```python
from build123d import *

# Parameters (mm, degrees)
F0_W     = 114.3
F0_H     = 76.2
F1_DEPTH = 25.4
F2_R     = 5.08
F3_T     = -3.81
F4_R     = 4.953
F5_DEPTH = 25.4
F7_DEPTH = 3.81


with BuildPart() as f1:
    # F0 (on Top) → F1 (new body)
    with BuildSketch(Plane.XY):
        with Locations((57.15, -38.1)):
            Rectangle(F0_W, F0_H)
    extrude(amount=F1_DEPTH)

    # F2
    f2_edges = [f1.edges().sort_by_distance(p)[0] for p in [
        (114.3, 0, 12.7),
        (114.3, -76.2, 12.7),
        (0, 0, 12.7),
        (0, -76.2, 12.7),
    ]]
    fillet(f2_edges, radius=F2_R)

    # F3
    f3_openings = [f1.faces().sort_by_distance(p)[0] for p in [
        (57.15, -38.1, 0),
    ]]
    offset(amount=F3_T, openings=f3_openings)

    # F4 (on face) → F5 (cut)
    with BuildSketch(Plane.YZ.offset(114.3)):
        with Locations((-25.4, 12.7)):
            Circle(F4_R)
    extrude(amount=-F5_DEPTH, mode=Mode.SUBTRACT)

    # F6 (on face) → F7 (join)
    with BuildSketch(Plane.XY.offset(25.4)):
        with BuildLine():
            Line((109.22, 3.937), (5.08, 3.937))
            ThreePointArc((5.08, 3.937), (-1.295982, 1.295982), (-3.937, -5.08))
            Line((-3.937, -5.08), (-3.937, -71.12))
            ThreePointArc((-3.937, -71.12), (-1.295982, -77.495982), (5.08, -80.137))
            Line((5.08, -80.137), (109.22, -80.137))
            ThreePointArc((109.22, -80.137), (115.595982, -77.495982), (118.237, -71.12))
            Line((118.237, -71.12), (118.237, -5.08))
            ThreePointArc((118.237, -5.08), (115.595982, 1.295982), (109.22, 3.937))
        make_face()
        with BuildLine():
            ThreePointArc((-0.127, -5.08), (1.398095, -1.398095), (5.08, 0.127))
            Line((5.08, 0.127), (109.22, 0.127))
            ThreePointArc((109.22, 0.127), (112.901905, -1.398095), (114.427, -5.08))
            Line((114.427, -5.08), (114.427, -71.12))
            ThreePointArc((114.427, -71.12), (112.901905, -74.801905), (109.22, -76.327))
            Line((109.22, -76.327), (5.08, -76.327))
            ThreePointArc((5.08, -76.327), (1.398095, -74.801905), (-0.127, -71.12))
            Line((-0.127, -71.12), (-0.127, -5.08))
        make_face(mode=Mode.SUBTRACT)
        with BuildLine():
            Line((109.22, 0.127), (5.08, 0.127))
            ThreePointArc((5.08, 0.127), (1.398095, -1.398095), (-0.127, -5.08))
            Line((-0.127, -5.08), (-0.127, -71.12))
            ThreePointArc((-0.127, -71.12), (1.398095, -74.801905), (5.08, -76.327))
            Line((5.08, -76.327), (109.22, -76.327))
            ThreePointArc((109.22, -76.327), (112.901905, -74.801905), (114.427, -71.12))
            Line((114.427, -71.12), (114.427, -5.08))
            ThreePointArc((114.427, -5.08), (112.901905, -1.398095), (109.22, 0.127))
        make_face()
        with BuildLine():
            ThreePointArc((5.08, -76.2), (1.487898, -74.712102), (0, -71.12))
            Line((0, -71.12), (0, -5.08))
            ThreePointArc((0, -5.08), (1.487898, -1.487898), (5.08, 0))
            Line((5.08, 0), (109.22, 0))
            ThreePointArc((109.22, 0), (112.812102, -1.487898), (114.3, -5.08))
            Line((114.3, -5.08), (114.3, -71.12))
            ThreePointArc((114.3, -71.12), (112.812102, -74.712102), (109.22, -76.2))
            Line((109.22, -76.2), (5.08, -76.2))
        make_face(mode=Mode.SUBTRACT)
        with BuildLine():
            Line((0, -5.08), (0, -71.12))
            ThreePointArc((0, -71.12), (1.487898, -74.712102), (5.08, -76.2))
            Line((5.08, -76.2), (109.22, -76.2))
            ThreePointArc((109.22, -76.2), (112.812102, -74.712102), (114.3, -71.12))
            Line((114.3, -71.12), (114.3, -5.08))
            ThreePointArc((114.3, -5.08), (112.812102, -1.487898), (109.22, 0))
            Line((109.22, 0), (5.08, 0))
            ThreePointArc((5.08, 0), (1.487898, -1.487898), (0, -5.08))
        make_face()
    extrude(amount=F7_DEPTH)


solid = f1.part
```
Read the model definition and answer for the solid it produces. Units are mm, in the model's axes. A direction names the side the tool comes from. Round coordinates to 2 decimals unless told otherwise and drop trailing zeros. Write each loop counter-clockwise with the first axis right and the second up, starting at its lowest first coordinate (ties: lowest second). Pieces come first, ordered by that corner, then holes. Notation, with made-up numbers: (12.25, 56) - (42.25, 56) arc R37 ccw to (42.25, 94) - close; hole circle Ø7 at (-13.5, 53). An arc over 180 degrees is marked (long way). One line per item, written item: value.
Q1. Straight lines are drawn through the part: line 1 (X direction, y = -17.5, z = 19.25); line 2 (Z direction, x = 113.15, y = -25.4); line 3 (Y direction, x = 64.5, z = 2.25). For each, find the intervals that lie inside material, in ascending order. Write a range as from..to.
The answers:
line 1: x = 0..3.81, 110.49..114.3
line 2: z = 0..7.75, 17.65..29.21
line 3: y = -76.2..-72.39, -3.81..0
Q2. Find section B-B (z = 12.7). Determine the outline of the cut face in (x, y).
The answers:
outline: (0, -71.12) arc R5.08 ccw to (5.08, -76.2) - (109.22, -76.2) arc R5.08 ccw to (114.3, -71.12) - (114.3, -30.35) - (110.49, -30.35) - (110.49, -71.12) arc R1.27 cw to (109.22, -72.39) - (5.08, -72.39) arc R1.27 cw to (3.81, -71.12) - (3.81, -5.08) arc R1.27 cw to (5.08, -3.81) - (109.22, -3.81) arc R1.27 cw to (110.49, -5.08) - (110.49, -20.45) - (114.3, -20.45) - (114.3, -5.08) arc R5.08 ccw to (109.22, 0) - (5.08, 0) arc R5.08 ccw to (0, -5.08) - close
Q3. Find section A-A (y = -25.4). Determine the outline of the cut face in (x, z).
The answers:
outline: (-3.94, 25.4) - (0, 25.4) - (0, 0) - (3.81, 0) - (3.81, 21.59) - (110.49, 21.59) - (110.49, 17.65) - (114.3, 17.65) - (114.3, 25.4) - (118.24, 25.4) - (118.24, 29.21) - (-3.94, 29.21) - close; (110.49, 0) - (114.3, 0) - (114.3, 7.75) - (110.49, 7.75) - close
Q4. Each of these flat-tipped pins is pushed along its axis until it touches: P1, Ø1, axis at x = 57, y = -62, coming from the -Z side; P2, Ø1, axis at y = -48, z = 5, coming from the -X side; P3, Ø11, axis at x = 36.5, z = 9.5, coming from the -Y side. Where does it stop, or does it pass through?
The answers:
P1: stops at z = 21.59
P2: stops at x = 0
P3: stops at y = -76.2
Q5. For a pull along Y with two mould halves and no side action, classify faces 4 (the flat face through (53, -75, 0)), 5 (the flat face through (110.49, -39, 11)), 6 (the cylindrical face through (115.525, -77.566, 27.278)) as pulls with the +Y half, pulls with the -Y half, needs draft (parallel to the pull), parting line crosses it, or undercut.
The answers:
face 4: needs draft
face 5: undercut
face 6: pulls with the -Y half
Q6. Which of the six approach directions +Z, -Z, +X, -X, +Y, -Y give full straight-line access (tool end or side, diameter ignored) to faces 1 (the cylindrical face through (1.449, -74.672, 12.878)), 2 (the cylindrical face through (112.772, -74.751, 12.878)), 3 (the flat face through (56, -72.39, 11))?
The answers:
face 1: -Z, -X, -Y
face 2: -Z, +X, -Y
face 3: -Z
Q7. Find section C-C (x = 102.5). Determine the outline of the cut face in (y, z).
The answers:
outline: (-80.14, 25.4) - (-76.2, 25.4) - (-76.2, 0) - (-72.39, 0) - (-72.39, 21.59) - (-3.81, 21.59) - (-3.81, 0) - (0, 0) - (0, 25.4) - (3.94, 25.4) - (3.94, 29.21) - (-80.14, 29.21) - close
Q8. Find section D-D (y = -59.5). Determine the outline of the cut face in (x, z).
The answers:
outline: (-3.94, 25.4) - (0, 25.4) - (0, 0) - (3.81, 0) - (3.81, 21.59) - (110.49, 21.59) - (110.49, 0) - (114.3, 0) - (114.3, 25.4) - (118.24, 25.4) - (118.24, 29.21) - (-3.94, 29.21) - close
